```python
from build123d import *

# Parameters (mm, degrees)
BOSS_EXTRUDE1_DEPTH = 3
FILLET1_R           = 4
FILLET2_R           = 1
FILLET3_R           = 7


with BuildPart() as part:
    # Sketch1 → Boss-Extrude1 (new body)
    with BuildSketch(Plane(origin=(0, 0, 0), x_dir=(1, 0, 0), z_dir=(0, 1, 0))):
        with BuildLine():
            Line((-1.5, 15.76), (-1.5, 0))
            ThreePointArc((-1.5, 0), (0, -1.5), (1.5, 0))
            Line((1.5, 0), (1.5, 15.76))
            Line((1.5, 15.76), (8.39, 15.76))
            Line((8.39, 15.76), (8.39, 0))
            ThreePointArc((8.39, 0), (9.89, -1.5), (11.39, 0))
            Line((11.39, 0), (11.39, 15.76))
            Line((11.39, 15.76), (20.345, 15.76))
            Line((20.345, 15.76), (18, -1.5))
            Line((18, -1.5), (24, -1.5))
            Line((24, -1.5), (26.209136732, 14.76))
            Line((26.209136732, 14.76), (29.439136732, 14.76))
            Line((29.439136732, 14.76), (27.375, -16.54))
            Line((27.375, -16.54), (19.725, -19.4))
            Line((19.725, -19.4), (20.405, -30.24))
            Line((20.405, -30.24), (17.97, -34.24))
            Line((17.97, -34.24), (11.39, -34.24))
            Line((11.39, -34.24), (11.39, -23.125))
            ThreePointArc((11.39, -23.125), (9.89, -21.625), (8.39, -23.125))
            Line((8.39, -23.125), (8.39, -34.24))
            Line((8.39, -34.24), (1.5, -34.24))
            Line((1.5, -34.24), (1.5, -23.125))
            ThreePointArc((1.5, -23.125), (0, -21.625), (-1.5, -23.125))
            Line((-1.5, -23.125), (-1.5, -34.24))
            Line((-1.5, -34.24), (-8.39, -34.24))
            Line((-8.39, -34.24), (-8.39, -23.125))
            ThreePointArc((-8.39, -23.125), (-9.89, -21.625), (-11.39, -23.125))
            Line((-11.39, -23.125), (-11.39, -34.24))
            Line((-11.39, -34.24), (-17.97, -34.24))
            Line((-17.97, -34.24), (-20.405, -30.24))
            Line((-20.405, -30.24), (-19.725, -19.4))
            Line((-19.725, -19.4), (-27.375, -16.54))
            Line((-27.375, -16.54), (-29.439136732, 14.76))
            Line((-29.439136732, 14.76), (-26.209136732, 14.76))
            Line((-26.209136732, 14.76), (-24, -1.5))
            Line((-24, -1.5), (-18, -1.5))
            Line((-18, -1.5), (-20.345, 15.76))
            Line((-20.345, 15.76), (-11.39, 15.76))
            Line((-11.39, 15.76), (-11.39, 0))
            ThreePointArc((-11.39, 0), (-9.89, -1.5), (-8.39, 0))
            Line((-8.39, 0), (-8.39, 15.76))
            Line((-8.39, 15.76), (-1.5, 15.76))
        make_face()
    extrude(amount=BOSS_EXTRUDE1_DEPTH)

    # Fillet1
    # the kernel refuses this fillet: 4 mm, written as the material it takes off along each edge
    with BuildSketch(Plane(origin=(-29.439136732, -10.340886874, -14.76), x_dir=(0.0658039254405357, 0, 0.9978325728280353), z_dir=(0, 1, 0))) as fillet1_piece_1:
        with BuildLine():
            CenterArc((4.136354749, 4), FILLET1_R, 191.20092555, 78.79907445)
            Line((0.212546679, 3.22299921), (0.134070518, 3.207459194))
            ThreePointArc((0.134070518, 3.207459194), (0.026446734, 1.616763919), (-0.079826606, 0.005264314))
            Line((-0.079826606, 0.005264314), (0, -0.08))
            Line((0, -0.08), (4.136354749, -0.08))
            Line((4.136354749, -0.08), (4.136354749, 0))
        make_face()
    extrude(amount=23.681773747, mode=Mode.SUBTRACT)
    with BuildSketch(Plane(origin=(29.439136732, -10.340886874, -14.76), x_dir=(-1, 0, 0), z_dir=(0, 1, 0))) as fillet1_piece_2:
        with BuildLine():
            CenterArc((4.263518671, 3.8641738), FILLET1_R, 176.226986492, 78.79907445)
            Line((0.27218838, 4.127389502), (0.192361774, 4.132653816))
            Line((0.192361774, 4.132653816), (-0.079826606, 0.005264314))
            Line((-0.079826606, 0.005264314), (0, -0.08))
            ThreePointArc((0, -0.08), (1.615, -0.08), (3.209329627, -0.077283476))
            Line((3.209329627, -0.077283476), (3.23, 0))
        make_face()
    extrude(amount=23.681773747, mode=Mode.SUBTRACT)

    # Fillet2
    fillet2_edges = [part.edges().sort_by_distance(p)[0] for p in [
        (18, 1.5, 1.5),
        (24, 1.5, 1.5),
        (-24, 1.5, 1.5),
        (-18, 1.5, 1.5),
    ]]
    fillet(fillet2_edges, radius=FILLET2_R)

    # Fillet3
    # the kernel refuses this fillet: 7 mm, written as the material it takes off along each edge
    with BuildSketch(Plane(origin=(-17.97, -9.834409558, 34.24), x_dir=(-0.5199808190603049, 0, -0.8541779368547132), z_dir=(0, 1, 0)), Plane(origin=(17.97, -9.834409558, 34.24), x_dir=(-1, 0, 0), z_dir=(0, 1, 0))) as fillet3_piece_1:
        with BuildLine():
            CenterArc((FILLET3_R * 0.561966260458, -FILLET3_R), FILLET3_R, 90, 58.669035113)
            Line((-FILLET3_R * 0.292211676397, -FILLET3_R * 0.48001918094), (0, 0))
            Line((0, 0), (FILLET3_R * 0.561966260458, 0))
        make_face()
    extrude(amount=22.668819116, mode=Mode.SUBTRACT)
    with BuildSketch(Plane(origin=(-20.405, -5.504377364, 30.24), x_dir=(0.06260756375388789, 0, -0.998038222194322), z_dir=(0, 1, 0)), Plane(origin=(20.405, -5.504377364, 30.24), x_dir=(-0.5199808190603047, 0, 0.8541779368547133), z_dir=(0, 1, 0))) as fillet3_piece_2:
        with BuildLine():
            CenterArc((FILLET3_R * 0.314535849376, -FILLET3_R), FILLET3_R, 90, 34.920461628)
            Line((-FILLET3_R * 0.257902882493, -FILLET3_R * 0.180052502744), (0, 0))
            Line((0, 0), (FILLET3_R * 0.314535849376, 0))
        make_face()
    extrude(amount=14.008754728, mode=Mode.SUBTRACT)
    with BuildSketch(Plane(origin=(-27.375, -11.305757053, 16.54), x_dir=(-0.06580392544053615, 0, -0.9978325728280353), z_dir=(0, 1, 0)), Plane(origin=(27.375, -11.305757053, 16.54), x_dir=(-0.9366809367224829, 0, 0.3501839841864447), z_dir=(0, 1, 0))) as fillet3_piece_3:
        with BuildLine():
            CenterArc((FILLET3_R * 0.646043260189, -FILLET3_R), FILLET3_R, 90, 65.728417673)
            Line((-FILLET3_R * 0.265564008034, -FILLET3_R * 0.588937731574), (0, 0))
            Line((0, 0), (FILLET3_R * 0.646043260189, 0))
        make_face()
    extrude(amount=25.611514107, mode=Mode.SUBTRACT)


solid = part.part
```
Read the model definition and answer for the solid it produces. Units are mm, in the model's axes. A direction names the side the tool comes from. Round coordinates to 2 decimals unless told otherwise and drop trailing zeros. Write each loop counter-clockwise with the first axis right and the second up, starting at its lowest first coordinate (ties: lowest second). Pieces come first, ordered by that corner, then holes. Notation, with made-up numbers: (60.5, 40.25) -> (108.5, 40.25) arc R8 cw to (108.5, 55.25) -> close; hole circle Ø7 at (55, 82.25). An arc over 180 degrees is marked (long way). Answer in a Markdown table with one row per item. Add a question column.
1) Consider line 1 (X direction, y = 2.45, z = 28.5); line 2 (X direction, y = 2.85, z = -9); line 3 (X direction, y = 0.95, z = -14). Determine where each line is inside the solid, lowest interval first.
2) Given P1, Ø1.5, axis at y = 1.5, z = 28.5, coming from the +X side; P2, Ø0.9, axis at y = 2, z = -6.5, coming from the +X side; P3, Ø1, axis at x = 15, y = 1, coming from the +Z side, each flat-ended and moving along its own axis, determine where each tip first touches the part or whether it passes through.
3) Find section A-A, the plane z = -11.5. Determine the outline of the cut face in (x, y).
4) Find section B-B, the plane z = 24.5. Determine the outline of the cut face in (x, y), and give its area (3 significant figures).
5) Find section C-C, the plane x = -9.89. Determine the outline of the cut face in (y, z) (3 decimals).
6) Determine the mould class of faces 1 (the face through (-17.184, 1.479, 33.492)), 2 (the face through (-20, 1.5, 23.8)), 3 (the face through (19.992, 1.479, 23.661)), 4 (the face through (11.39, 1, 29)) for opening direction Z: pulls with the +Z half, pulls with the -Z half, needs draft (parallel to the pull), parting line crosses it, or undercut.
7) Which of the six approach directions +Z, -Z, +X, -X, +Y, -Y give full straight-line access (tool end or side, diameter ignored) to faces 5 (the face through (8.39, 1, 29)), 6 (the face through (26.27, 1.48, 15.79)), 7 (the face through (11.39, 1, -8))?
Findings below:
| question | item | result |
|---|---|---|
| 1 | line 1 | -20.28 to -11.39, -8.39 to -1.5, 1.5 to 8.39, 11.39 to 20.28 |
| 1 | line 2 | -29.06 to -25.43, -19.43 to -11.39, -8.39 to -1.5, 1.5 to 8.39, 11.39 to 19.43, 25.43 to 29.06 |
| 1 | line 3 | -27.7 to -26.11, -20.11 to -11.39, -8.39 to -1.5, 1.5 to 8.39, 11.39 to 20.11, 26.11 to 27.7 |
| 2 | P1 | x = 20.28 |
| 2 | P2 | x = 28.92 |
| 2 | P3 | z = 34.22 |
| 3 | outline | (-29.13, 0) -> (-25.77, 0) -> (-25.77, 3) -> (-29.13, 3) -> close; (-19.77, 0) -> (-11.39, 0) -> (-11.39, 3) -> (-19.77, 3) -> close; (-8.39, 0) -> (-1.5, 0) -> (-1.5, 3) -> (-8.39, 3) -> close; (1.5, 0) -> (8.39, 0) -> (8.39, 3) -> (1.5, 3) -> close; (11.39, 0) -> (19.77, 0) -> (19.77, 3) -> (11.39, 3) -> close; (25.77, 0) -> (29.13, 0) -> (29.13, 3) -> (25.77, 3) -> close |
| 4 | outline | (-20.04, 0) -> (-11.39, 0) -> (-11.39, 3) -> (-20.04, 3) -> close; (-8.39, 0) -> (-1.5, 0) -> (-1.5, 3) -> (-8.39, 3) -> close; (1.5, 0) -> (8.39, 0) -> (8.39, 3) -> (1.5, 3) -> close; (11.39, 0) -> (20.04, 0) -> (20.04, 3) -> (11.39, 3) -> close |
| 4 | area | 93.3 mm² |
| 5 | outline | (0, 1.5) -> (3, 1.5) -> (3, 21.625) -> (0, 21.625) -> close |
| 6 | face 1 | pulls with the +Z half |
| 6 | face 2 | undercut |
| 6 | face 3 | undercut |
| 6 | face 4 | needs draft |
| 7 | face 5 | +Z, +Y, -Y |
| 7 | face 6 | +Z, +X, +Y, -Y |
| 7 | face 7 | -Z, +Y, -Y |
